CAD build for the part. Positions are in the model's coordinates, mm. A direction names the side the tool comes from. Give positions to 0.01 mm unless a question says otherwise; leave off trailing zeros. Write each loop counter-clockwise with the first axis right and the second up, starting at its lowest first coordinate (ties: lowest second). Pieces come first, ordered by that corner, then holes. Notation, with made-up numbers: M 13,-25 L 51,-25 A16 cw 51,-11 Z; hole C 17.25,-24 d1. An arc over 180 degrees is marked long. One line per question, with ' | ' between items. Start each with the question number.
1. Cut at C-C, the plane y = -9.5. Count the separate pieces of the cut face and the enclosed holes in it, then the cut area to 3 significant figures.
2. Cut at D-D, the plane z = 43. Write the cut outline in (x, y), then the cut area to 3 significant figures.
3. Flat gauge pins, fed straight in: pin 1 (1.6 mm diameter, centred on x = 58, z = 1, fed in from -Y); pin 2 (2.5 mm diameter, centred on x = 59, z = 8.5, fed in from +Y); pin 3 (1 mm diameter, centred on x = 41, z = -43.5, fed in from -Y). Where does each tip first touch, or does it go through?
4. Wall check: L1, parallel to X at y = -3.75, z = 10.5; L2, parallel to Z at x = 17, y = -1 (3 decimals); L3, parallel to Z at x = 55.5, y = -9.5 (3 decimals). Give the ranges that are in metal, low to high.
5. Cut at A-A, the plane z = 8.5. Write the cut outline in (x, y).
6. Pull direction Z, two halves, no side cores. Call faces 5 (the face through (-21, -10, -37)), 6 (the face through (67, -6, -1)), 7 (the face through (-1, -6, -51)): released by +Z, released by -Z, zero draft, split by the parting line, or undercut.
7. Cut at B-B, the plane x = -51. Write the cut outline in (y, z) (3 decimals), then the cut area to 3 significant figures.
8. Which spindle directions (+Z, -Z, +X, -X, +Y, -Y) get a long thin tool onto all of the face, cutting with end or side? Do faces 1 (the face through (-21, -12.7, -20)), 2 (the face through (-21, -10, 2.625)), 3 (the face through (-57, -6.35, -41)), 4 (the face through (-59.42, -1.6, 37.89)). Say none if no direction does.
```python
from build123d import *

# Parameters (mm, degrees)
F0_W      = 134
F0_H      = 102
F1_DEPTH  = 12.7
F2_W      = 29.5
F2_H      = 79.6
F3_DEPTH  = 12.7
F4_W      = 117
F4_H      = 7.5
F4_W_2    = 134
F4_H_2    = 5.25
F5_DEPTH  = 6.35
F8_DEPTH  = 3.25
F9_W      = 29.5
F9_H      = 4.7
F10_DEPTH = 3.3


with BuildPart() as f1:
    # F0 (on Front) → F1 (new body)
    with BuildSketch(Plane.XZ):
        Rectangle(F0_W, F0_H)
    extrude(amount=F1_DEPTH)

    # F2 (on face) → F3 (cut)
    with BuildSketch(Plane.XZ.offset(12.7)):
        with Locations((-1.25, 0)):
            Rectangle(F2_W, F2_H)
        Polygon((53, 39.8), (23.5, 39.8), (23.5, -39.8), (53, -39.8), (53, -16.022205), align=None)
        with Locations((-40.75, 0)):
            Rectangle(F2_W, F2_H)
    extrude(amount=-F3_DEPTH, mode=Mode.SUBTRACT)

    # F4 (on face) → F5 (cut)
    with BuildSketch(Plane.XZ.offset(12.7)):
        with Locations((0, 40.75)):
            Rectangle(F4_W, F4_H)
        Rectangle(F4_W_2, F4_H_2)
        with Locations((0, -40.75)):
            Rectangle(F4_W, F4_H)
    extrude(amount=-F5_DEPTH, mode=Mode.SUBTRACT)

    # F7 (on face) → F8 (cut)
    with BuildSketch(Plane(origin=(0, 0, 0), x_dir=(-1, 0, 0), z_dir=(0, 1, 0))):
        Polygon((56.5, 41.125), (-62, 41.125), (-62, -41.125), (56.5, -41.125), (62.25, -34.75), (62.25, 34.75), align=None)
    extrude(amount=-F8_DEPTH, mode=Mode.SUBTRACT)

    # F9 (on face) → F10 (cut)
    with BuildSketch(Plane.XZ.offset(6.35)):
        with Locations((-1.25, 42.15)):
            Rectangle(F9_W, F9_H)
        with Locations((38.25, 42.15)):
            Rectangle(F9_W, F9_H)
        with Locations((-40.75, 42.15)):
            Rectangle(F9_W, F9_H)
        with Locations((-40.75, -42.15)):
            Rectangle(F9_W, F9_H)
        with Locations((-1.25, -42.15)):
            Rectangle(F9_W, F9_H)
        with Locations((38.25, -42.15)):
            Rectangle(F9_W, F9_H)
    extrude(amount=-F10_DEPTH, mode=Mode.SUBTRACT)


solid = f1.part
```
Here are the results:
1) separate pieces: 6 | enclosed holes: 0 | area: 5,130 mm^2
2) outline: M -67,-12.7 L -58.5,-12.7 L -58.5,-6.35 L -55.5,-6.35 L -55.5,-3.05 L -26,-3.05 L -26,-6.35 L -16,-6.35 L -16,-3.05 L 13.5,-3.05 L 13.5,-6.35 L 23.5,-6.35 L 23.5,-3.05 L 53,-3.05 L 53,-6.35 L 58.5,-6.35 L 58.5,-12.7 L 67,-12.7 L 67,0 L -67,0 Z | area: 667 mm^2
3) pin 1: y = -6.35 | pin 2: y = -3.25 | pin 3: y = -3.05
4) L1: -67 to -55.5, -26 to -16, 13.5 to 23.5, 53 to 67 | L2: -51 to -41.125, 41.125 to 51 | L3: -51 to -44.5, -37 to -2.625, 2.625 to 37, 44.5 to 51
5) outline: M -67,-12.7 L -55.5,-12.7 L -55.5,-3.25 L -62.25,-3.25 L -62.25,0 L -67,0 Z; M -26,-12.7 L -16,-12.7 L -16,-3.25 L -26,-3.25 Z; M 13.5,-12.7 L 23.5,-12.7 L 23.5,-3.25 L 13.5,-3.25 Z; M 53,-12.7 L 67,-12.7 L 67,0 L 62,0 L 62,-3.25 L 53,-3.25 Z
6) face 5: undercut | face 6: zero draft | face 7: released by -Z
7) outline: M -12.7,-51 L 0,-51 L 0,-41.125 L -3.05,-41.125 L -3.05,-44.5 L -12.7,-44.5 Z; M -12.7,44.5 L -3.05,44.5 L -3.05,41.125 L 0,41.125 L 0,51 L -12.7,51 Z | area: 186 mm^2
8) face 1: +Z, -Z, +X, -X, -Y | face 2: +X, -X, -Y | face 3: -Y | face 4: +Y
